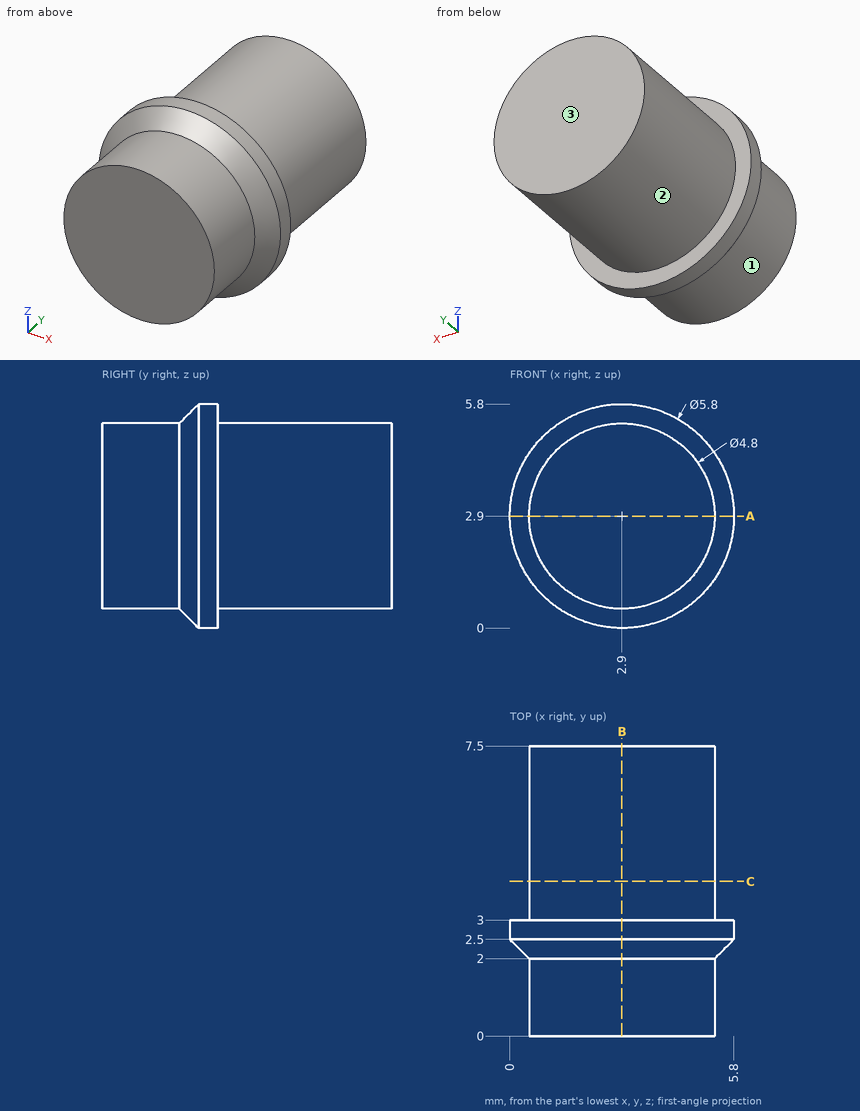
Input: dimensioned drawing with shaded views. Units: mm. Origin: part minimum x, y, z. A direction names the side the tool comes from. Round coordinates to 2 decimals unless told otherwise and drop trailing zeros. Loops run counter-clockwise (first coordinate to the right, second up) from the corner with the lowest first, then second, coordinate; pieces in that order, holes last. Notation, with made-up numbers: (-33.5, 42) -> (-17.5, 42) arc R30 ccw to (-17.5, 68) -> close; hole circle Ø3 at (17, 83.5). An arc over 180 degrees is marked (long way). Use one line per item in the form item = value. Start each with the question number.
1) Section C-C on y = 4. Output: boundary loops of the cut face in (x, z), then the cut area to 3 significant figures.
2) Section B-B on x = 2.9. Output: boundary loops of the cut face in (y, z).
3) Access query for the marked faces 1, 2 and 3. Directions: +Z, -Z, +X, -X, +Y, -Y. A direction counts if a zero-diameter tool reaches every point of the face in a straight line with its end or side. Return the directions, or none.
4) Section A-A on z = 2.9. Output: boundary loops of the cut face in (x, y).
5) Line query: L1, parallel to X at y = 5.5, z = 3; L2, parallel to Z at x = 4.9, y = 5.25; L3, parallel to Z at x = 3.25, y = 1.75. Output: solid intervals per line, ascending.
6) First-contact query: P1, Ø1.5, axis at x = 1.5, y = 6.5, coming from the +Z side. Flat tip, straight axial feed; report the tip coordinate or a pass-through.
Response:
q1.outline = circle Ø4.8 at (2.9, 2.9)
q1.area = 18.1 mm^2
q2.outline = (0, 0.5) -> (2, 0.5) -> (2.5, 0) -> (3, 0) -> (3, 0.5) -> (7.5, 0.5) -> (7.5, 5.3) -> (3, 5.3) -> (3, 5.8) -> (2.5, 5.8) -> (2, 5.3) -> (0, 5.3) -> close
q3.face_1 = -Y
q3.face_2 = +Y
q3.face_3 = +Z, -Z, +X, -X, +Y
q4.outline = (0, 2.5) -> (0.5, 2) -> (0.5, 0) -> (5.3, 0) -> (5.3, 2) -> (5.8, 2.5) -> (5.8, 3) -> (5.3, 3) -> (5.3, 7.5) -> (0.5, 7.5) -> (0.5, 3) -> (0, 3) -> close
q5.L1 = 0.5 to 5.3
q5.L2 = 1.57 to 4.23
q5.L3 = 0.53 to 5.27
q6.P1 = 5.21
